Solid Edge part; units mm, degrees
sketch "Sketch1" plane through (0, 0, 0) normal (0, -1, 0) x (1, 0, 0)
  circle A0 centre (0, 0) radius 1.5
extrude "Protrusion1" add sketch "Sketch1" against normal blind 12
sketch "Sketch2" plane through (0, 12, 0) normal (0, 1, 0) x (1, 0, 0)
  circle A0 centre (0, 0) radius 2.75
extrude "ExtrudedProtrusion_2" add sketch "Sketch2" along normal blind 2.52
sketch "Sketch3" plane through (0, 14.52, 0) normal (0, 1, 0) x (-1, 0, 0)
  line L0 (0.7217, 1.25) -> (-0.7217, 1.25)
  line L1 (-0.7217, 1.25) -> (-1.4434, 0)
  line L2 (-1.4434, 0) -> (-0.7217, -1.25)
  line L3 (-0.7217, -1.25) -> (0.7217, -1.25)
  line L4 (0.7217, -1.25) -> (1.4434, 0)
  line L5 (1.4434, 0) -> (0.7217, 1.25)
extrude "Cutout1" cut sketch "Sketch3" against normal blind 1.3
chamfer "Chamfer1" distance 0.15 angle 45 1 edges at (-2.75, 14.52, 0)
properties material "Steel"
CAD build for the part. Positions are in the model's coordinates, mm. A direction names the side the tool comes from. Give positions to 0.01 mm unless a question says otherwise; leave off trailing zeros. Order: outer loops, then holes, each group sorted by start corner. A loop starts at its lowest first (then second) coordinate and runs counter-clockwise, first axis right, second up. Notation, with made-up numbers: (83.25, -20.5) -> (123.25, -20.5) arc R29 cw to (123.25, 17.5) -> close; hole circle Ø4 at (86, -8). An arc over 180 degrees is marked (long way). Return JSON: item names as keys, results as strings.
Q1. Drill centre lines: line 1 (Y direction, x = 0.2, z = -2.4); line 2 (X direction, y = 13.75, z = -1.15); line 3 (Z direction, x = 0.05, y = 11.25). Where is each one in solid material? Low to high.
Working result:
{"line 1": "12 to 14.52", "line 2": "-2.5 to -0.78, 0.78 to 2.5", "line 3": "-1.5 to 1.5"}
Q2. Saw through at A-A (x = 0). Write the cut outline in (y, z).
Working result:
{"outline": "(0, -1.5) -> (12, -1.5) -> (12, -2.75) -> (14.37, -2.75) -> (14.52, -2.6) -> (14.52, -1.25) -> (13.22, -1.25) -> (13.22, 1.25) -> (14.52, 1.25) -> (14.52, 2.6) -> (14.37, 2.75) -> (12, 2.75) -> (12, 1.5) -> (0, 1.5) -> close"}
Q3. Saw through at B-B (y = 11.75). Write the cut outline in (x, z), then the cut area to 3 significant figures.
Working result:
{"outline": "circle Ø3 at (0, 0)", "area": "7.07 mm²"}
Q4. Which spindle directions (+Z, -Z, +X, -X, +Y, -Y) get a long thin tool onto all of the face, cutting with end or side? Do faces 4 (the face through (-1.5, 5.92, 0.07)), 5 (the face through (0, 14, -1.25)), 6 (the face through (0, 0, 0)). Say none if no direction does.
Working result:
{"face 4": "-Y", "face 5": "+Y", "face 6": "+Z, -Z, +X, -X, -Y"}
Q5. Mould opens along X. For faces 1 (the face through (-1.1, 14.52, 1.1)), 2 (the face through (-0.596, 13.168, -2.685)), 3 (the face through (-1.088, 13.879, 0.616)) say: pulls with the +X half, pulls with the -X half, needs draft (parallel to the pull), parting line crosses it, or undercut.
Working result:
{"face 1": "needs draft", "face 2": "parting line crosses it", "face 3": "undercut"}
Q6. Flat gauge pins, fed straight in: pin 1 (1 mm diameter, centred on y = 12.5, z = 1, fed in from -X); pin 2 (0.8 mm diameter, centred on x = 0, z = -0.5, fed in from +Y); pin 3 (0.6 mm diameter, centred on x = -0.5, y = 14, fed in from +Z). Where does each tip first touch, or does it go through?
Working result:
{"pin 1": "x = -2.7", "pin 2": "y = 13.22", "pin 3": "z = 2.74"}
